Autodesk Inventor part; units mm, degrees
ref_plane "Work Plane1" through (0, 0, 0) normal (0.7071, 0, -0.7071) x (0, 1, 0)
ref_plane "YZ Plane" through (0, 0, 0) normal (1, 0, 0) x (0, 1, 0)
ref_plane "XZ Plane" through (0, 0, 0) normal (0, 1, 0) x (-1, 0, 0)
sketch "Sketch1" plane through (0, 0, 0) normal (0, 1, 0) x (-1, 0, 0)
  point P0 (0, 0)
sketch "Sketch2" plane through (0, 0, 0) normal (0, 1, 0) x (-1, 0, 0)
  line L0 (120, 120) -> (-120, 120)
  line L1 (-120, 120) -> (-120, -120)
  line L2 (-120, -120) -> (120, -120)
  line L3 (120, -120) -> (120, 120)
  circle A0 centre (0, 0) radius 37.5
  dimension "d0" = 240
  dimension "d1" = 240
  dimension "d3" = 120
  dimension "d4" = 120
  dimension "d5" = 75
extrude "Extrusion1" add sketch "Sketch2" along normal blind 100
fillet "Fillet1" radius 6 1 edges at (-120, 50, -120)
fillet "Fillet2" radius 6 1 edges at (120, 50, -120)
fillet "Fillet3" radius 6 1 edges at (120, 50, 120)
fillet "Fillet4" radius 6 1 edges at (-120, 50, 120)
sketch "Sketch3" plane through (0, 100, 0) normal (0, 1, 0) x (1, 0, 0)
  line L0 (0, 0) -> (75, 0) construction
  point P0 (-75, 0)
  point P1 (0, 75)
  point P2 (0, 75)
  point P3 (0, -75)
  point P4 (-53.033, 53.033)
  point P5 (-53.033, 53.033)
  point P6 (53.033, 53.033)
  point P7 (53.033, -53.033)
  point P8 (-53.033, -53.033)
  dimension "d14" = 53.033
  dimension "d15" = 53.033
  dimension "d16" = 53.033
  dimension "d17" = 53.033
  dimension "d18" = 53.033
  dimension "d19" = 53.033
hole "Hole1" at (-75, 100, 0) at (75, 100, 0) at (0, 100, -75) at (0, 100, 75) at (-53.033, 100, -53.033) at (53.033, 100, -53.033) at (53.033, 100, 53.033) at (-53.033, 100, 53.033) direction (0, -1, 0) diameter 6 depth 10 tip angle 118
sketch "Sketch4" plane through (0, 100, 0) normal (0, 1, 0) x (1, 0, 0)
  point P0 (0, 0)
  point P1 (-112.5, 112.5)
  point P2 (-112.5, -112.5)
  point P3 (112.5, -112.5)
  point P4 (112.5, 112.5)
  dimension "d34" = 112.5
  dimension "d35" = 112.5
hole "Hole2" at (-112.5, 100, -112.5) at (-112.5, 100, 112.5) at (112.5, 100, 112.5) at (112.5, 100, -112.5) direction (0, -1, 0) diameter 8 end through all
sketch "Sketch5" plane through (0, 100, 0) normal (0, 1, 0) x (1, 0, 0)
  line L0 (95, 120) -> (120, 95)
  line L1 (120, -114) -> (120, 114)
  line L2 (95, 120) -> (130.3553, 120) construction
  line L3 (114, 120) -> (-114, 120)
  line L4 (-95, 120) -> (-120, 95)
  line L5 (-120, 114) -> (-120, -114)
  line L6 (-95, 120) -> (-59.6447, 120) construction
  line L7 (95, 120) -> (120, 120)
  line L8 (120, 120) -> (120, 95)
  line L9 (-95, 120) -> (-120, 120)
  line L10 (-120, 120) -> (-120, 95)
  point P0 (0, 0)
  dimension "d36" = 45
  dimension "d38" = 135
extrude "Extrusion2" cut sketch "Sketch5" against normal blind 87 contours L3 L7 L8 L1 L0
sketch "Sketch6" plane through (0, 100, 0) normal (0, 1, 0) x (1, 0, 0)
  line L0 (114, 120) -> (-114, 120)
  line L1 (-95, 120) -> (-120, 95)
  line L2 (-120, 114) -> (-120, -114)
  line L3 (-95, 120) -> (-59.6447, 120) construction
  line L4 (-95, 120) -> (-120, 120)
  line L5 (-120, 120) -> (-120, 95)
  point P0 (0, 0)
  dimension "d41" = 135
extrude "Extrusion3" cut sketch "Sketch6" against normal blind 87
sketch "Sketch7" plane through (0, 100, 0) normal (0, 1, 0) x (1, 0, 0)
  line L0 (120, -114) -> (120, 95)
  line L1 (120, -95) -> (95, -120)
  line L2 (-114, -120) -> (114, -120)
  line L3 (120, -95) -> (155.3553, -95) construction
  line L4 (120, -95) -> (120, -120)
  line L5 (120, -120) -> (95, -120)
  point P0 (0, 0)
  dimension "d44" = 135
extrude "Extrusion4" cut sketch "Sketch7" against normal blind 87
sketch "Sketch8" plane through (0, 100, 0) normal (0, 1, 0) x (1, 0, 0)
  line L0 (-120, 95) -> (-120, -114)
  line L1 (-120, -95) -> (-95, -120)
  line L2 (-114, -120) -> (95, -120)
  line L3 (-120, -95) -> (-84.6447, -95) construction
  line L4 (-95, -120) -> (-120, -120)
  line L5 (-120, -120) -> (-120, -95)
  point P0 (0, 0)
  dimension "d47" = 45
extrude "Extrusion5" cut sketch "Sketch8" against normal blind 87
sketch "Sketch9" plane through (0, 100, 0) normal (0, 1, 0) x (1, 0, 0)
  circle A0 centre (0, 0) radius 116.75
  line L0 (120, 120) -> (-120, 120)
  line L1 (-120, 120) -> (-120, -120)
  line L2 (-120, -120) -> (120, -120)
  line L3 (120, -120) -> (120, 120)
  dimension "d50" = 233.5
  dimension "d53" = 240
  dimension "d54" = 240
extrude "Extrusion6" cut sketch "Sketch9" against normal blind 3
ref_plane "Work Plane1" through (0, 0, 0) normal (0.7071, 0, -0.7071) x (0, 1, 0)
sketch "Sketch10" plane through (0, 0, 0) normal (0.7071, 0, -0.7071) x (0, 1, 0)
  line L0 (97, 116.75) -> (135.5145, 116.75) construction
  line L1 (97, -116.75) -> (97, 116.75)
  line L2 (97, 116.75) -> (151.2428, 116.75) construction
  line L3 (-153.1261, 0) -> (197.3136, 0)
  arc A0 (97, 120) -> (84.2851, 167.4528) centre (-101.0801, 92.3545) ccw
  line L4 (97, 120) -> (84.2851, 167.4528) construction
  line L5 (97, 120) -> (146.1267, 120) construction
  line L6 (84.2851, 167.4528) -> (97, 167.4528)
  line L7 (97, 167.4528) -> (97, 120)
  line L8 (97, 17.6777) -> (97, 152.028)
  line L9 (100, -116.75) -> (100, 116.75)
  point P0 (0, 0)
  dimension "d62" = 105
  dimension "d63" = 200
  dimension "d64" = 120
  dimension "d65" = 3
revolve "Revolution1" cut sketch "Sketch10" angle 360 about axis through (0, -10, 0) along (0, 1, 0)
sketch "Sketch11" plane through (0, 0, 0) normal (0.7071, 0, -0.7071) x (0, 1, 0)
  line L0 (97, -116.75) -> (97, 116.75)
  line L1 (97, 116.75) -> (100, 110.3165)
  line L2 (100, -116.75) -> (100, 116.75)
  line L3 (97, 116.75) -> (104.0986, 116.75) construction
  line L4 (100, 110.3165) -> (100, 116.75)
  line L5 (100, 116.75) -> (97, 116.75)
  line L6 (-21.7182, 0) -> (130.3093, 0)
  point P0 (0, 0)
  dimension "d66" = 65
revolve "Revolution2" cut sketch "Sketch11" angle 360 about axis through (0, -10, 0) along (0, 1, 0) contours L5 L2 L1
properties part number "DT240" material "Aluminum 6061"
Can you work these out from the model? Positions are in its coordinate system, mm. A direction names the side the tool comes from. Round coordinates to 2 decimals unless told otherwise and drop trailing zeros. Loops run counter-clockwise (first coordinate to the right, second up) from the corner with the lowest first, then second, coordinate; pieces in that order, holes last. Notation, with made-up numbers: M 32,87 L 58,87 A11 ccw 58,96 Z; hole C 7,47.5 d8. An arc over 180 degrees is marked long. Answer in a Markdown table with one row per item.
1. If we section it at A-A, the plane y = 37: Please give me the cut outline in (x, z).
Established:
| item | result |
|---|---|
| outline | M -120,-95 L -95,-120 L 95,-120 L 120,-95 L 120,95 L 95,120 L -95,120 L -120,95 Z; hole C 0,0 d75 |
2. Thinking about a two-plate mould opening in Z: for faces 6 (the face through (1.8, 94.9, 72.6)), 7 (the face through (-120, 48, -2)), 8 (the face through (105.583, 99.812, -33.331)), 9 (the face through (-53.233, 88.51, 53.514)), which applies, pulls with the +Z half, pulls with the -Z half, needs draft (parallel to the pull), parting line crosses it, or undercut?
Established:
| item | result |
|---|---|
| face 6 | undercut |
| face 7 | needs draft |
| face 8 | parting line crosses it |
| face 9 | undercut |
3. I'm going to push flat-ended pins straight in: pin 1 Ø1 at (x, z) = (40.5, -13) entering from -Y; pin 2 Ø20 at (x, z) = (-113.5, -104) entering from +Y; pin 3 Ø7.5 at (x, z) = (-109.5, 106) entering from +Y; pin 4 Ø13 at (x, z) = (112.5, 112.5) entering from +Y. Where does each tip first touch, or does it pass through?
Established:
| item | result |
|---|---|
| pin 1 | y = 0 |
| pin 2 | y = 92.15 |
| pin 3 | y = 90.83 |
| pin 4 | y = 13 |
4. Please list where these lines run through material, in increasing order: line 1 (Z direction, x = 112, y = 9); line 2 (X direction, y = 5.25, z = 112.5); line 3 (X direction, y = 24.5, z = 32). Write a range as from..to.
Established:
| item | result |
|---|---|
| line 1 | -120..-116.47, -108.53..108.53, 116.47..120 |
| line 2 | -120..-116.5, -108.5..108.5, 116.5..120 |
| line 3 | -120..-19.55, 19.55..120 |
5. On a 3-axis mill with a long thin cutter (end or side, diameter ignored), from which of +Z, -Z, +X, -X, +Y, -Y can I reach the whole of each face in a straight line? I mean faces 1 (the face through (28, 0, 28)), 2 (the face through (-110, 13, -108)), 3 (the face through (-50.104, 94.93, -53.683)), 4 (the face through (118.196, 6.591, 118.289)), 5 (the face through (-108, 52, 107)). Say none if no direction works.
Established:
| item | result |
|---|---|
| face 1 | +Z, -Z, +X, -X, -Y |
| face 2 | -Z, -X, +Y |
| face 3 | +Y |
| face 4 | +Z, +X, +Y, -Y |
| face 5 | +Z, -X, +Y |
